```python
from build123d import *

# Parameters (mm, degrees)
F0_W      = 6
F0_H      = 50
F1_DEPTH  = 6
F2_W      = 4
F2_H      = 4
F3_DEPTH  = 5
F5_DEPTH  = 1
F7_DEPTH  = 1
F8_DEPTH  = 4
F10_DEPTH = 25
F11_W     = 1
F11_H     = 4
F12_DEPTH = 25
F13_DEPTH = 15
F14_DEPTH = 15
F16_DEPTH = 1
F18_DEPTH = 1
F20_DEPTH = 4
F21_DEPTH = 1.333
F22_R     = 0.8
F23_SCALE = 0.8


with BuildPart() as f1:
    # F0 (on Top) → F1 (new body)
    with BuildSketch(Plane.XY):
        Rectangle(F0_W, F0_H)
    extrude(amount=F1_DEPTH)

    # F2 (on face) → F3 (join)
    with BuildSketch(Plane.XZ.offset(25)):
        with Locations((0, 2)):
            Rectangle(F2_W, F2_H)
    extrude(amount=F3_DEPTH)

    # F4 (on face) → F5 (cut)
    with BuildSketch(Plane(origin=(-3, 0, 0), x_dir=(0, -1, 0), z_dir=(-1, 0, 0))):
        Polygon((-25, 6), (-25, 0), (-23, 0), align=None)
    extrude(amount=-F5_DEPTH, mode=Mode.SUBTRACT)

    # F6 (on face) → F7 (cut)
    with BuildSketch(Plane.YZ.offset(3)):
        Polygon((23, 0), (25, 0), (25, 6), align=None)
    extrude(amount=-F7_DEPTH, mode=Mode.SUBTRACT)

    # F8 (add): a face of the model
    f8_faces = [f1.faces().sort_by_distance(p)[0] for p in [
        (0, 25, 3),
    ]]
    extrude(f8_faces, amount=F8_DEPTH)

    # F9 (on face) → F10 (cut)
    with BuildSketch(Plane.YZ.offset(2)):
        Polygon((26.5, 4), (26.5, 0), (29, 0), (29, 6), (25, 6), (24.3333333333, 4), align=None)
    extrude(amount=-F10_DEPTH, mode=Mode.SUBTRACT)

    # F11 (on face) → F12 (cut)
    with BuildSketch(Plane(origin=(-2, 0, 0), x_dir=(0, -1, 0), z_dir=(-1, 0, 0))):
        with Locations((29.5, 2)):
            Rectangle(F11_W, F11_H)
    extrude(amount=-F12_DEPTH, mode=Mode.SUBTRACT)

    # F13 (cut): a face of the model
    f13_faces = [f1.faces().sort_by_distance(p)[0] for p in [
        (-2.5, -25, 0.0848528137),
    ]]
    extrude(f13_faces, amount=-F13_DEPTH, mode=Mode.SUBTRACT)

    # F14 (cut): a face of the model
    f14_faces = [f1.faces().sort_by_distance(p)[0] for p in [
        (0, -29, 2),
    ]]
    extrude(f14_faces, amount=-F14_DEPTH, mode=Mode.SUBTRACT)

    # F15 (on face) → F16 (cut)
    with BuildSketch(Plane.YZ.offset(3)):
        Polygon((23, 0), (25, 6), (21, 6), align=None)
    extrude(amount=-F16_DEPTH, mode=Mode.SUBTRACT)

    # F17 (on face) → F18 (cut)
    with BuildSketch(Plane(origin=(-3, 0, 0), x_dir=(0, -1, 0), z_dir=(-1, 0, 0))):
        Polygon((-21, 6), (-25, 6), (-23, 0), align=None)
    extrude(amount=-F18_DEPTH, mode=Mode.SUBTRACT)

    # F19 (on face) → F20 (cut)
    with BuildSketch(Plane(origin=(-2, 0, 0), x_dir=(0, -1, 0), z_dir=(-1, 0, 0))):
        Polygon((-25, 6), (-24.3333333333, 4), (-21.6666666667, 4), (-21, 6), align=None)
    extrude(amount=-F20_DEPTH, mode=Mode.SUBTRACT)

    # F21 (cut): a face of the model
    f21_faces = [f1.faces().sort_by_distance(p)[0] for p in [
        (0, 26.5, 2),
    ]]
    extrude(f21_faces, amount=-F21_DEPTH, mode=Mode.SUBTRACT)

    # F22
    f22_edges = [f1.edges().sort_by_distance(p)[0] for p in [
        (3, 5.5, 6),
        (3, 6.5, 0),
        (-3, 5.5, 6),
        (-3, 6.5, 0),
    ]]
    fillet(f22_edges, radius=F22_R)


with BuildPart() as f1_1:
    # F23: moved
    add(f1.part.scale(F23_SCALE))


solid = f1_1.part
```
Can you work these out from the model? Positions are in its coordinate system, mm. A direction names the side the tool comes from. Coordinates: 2 decimals unless noted, no trailing zeros. Loops run counter-clockwise (first coordinate to the right, second up) from the corner with the lowest first, then second, coordinate; pieces in that order, holes last. Notation, with made-up numbers: (87, -21) -> (92, -21) arc R32 ccw to (92, 6) -> close; hole circle Ø6 at (15.5, -10.5). An arc over 180 degrees is marked (long way). Put each result on its own line as item: value. Start each with the question number.
Q1. I'm going to push flat-ended pins straight in: P1, Ø0.8, axis at x = 0, y = 19.5, coming from the +Z side; P2, Ø1.4, axis at y = 18.5, z = 1.5, coming from the +X side; P3, Ø2.5, axis at y = -9.5, z = 2, coming from the -X side; P4, Ø2.5, axis at y = -10, z = 1, coming from the +X side. Where does each tip first touch, or does it pass through?
Q2. I want a section at B-B (z = 2.4). Write out the boundary of the cut face in (x, y), plus the area to 3 significant figures.
Q3. I want a section at A-A (y = 16.5). Write out the boundary of the cut face in (x, z), plus the area to 3 significant figures.
Q4. I want a section at C-C (x = 0.85). Write out the boundary of the cut face in (y, z), plus the area to 3 significant figures.
Q5. If I drill on line 1 (X direction, y = 2, z = 4.25); line 2 (Z direction, x = 1.1, y = -8.5); line 3 (Z direction, x = -1.8, y = 11.5), over which ranges is the centre line in solid material (lowest first)? Write a range as [from, to].
Q6. For faces 1 (the face through (0, -10, 3.2)), 2 (the face through (0, 19, 3.2)), 3 (the face through (1.6, -10, 2)), which set-ups out of +Z, -Z, +X, -X, +Y, -Y let a thin tool reach every point of the face, with its end or its side?
Taken from the geometry:
1. P1: stops at z = 3.2
1. P2: stops at x = 2.4
1. P3: stops at x = -1.6
1. P4: stops at x = 1.6
2. outline: (-2.4, -8) -> (-1.6, -8) -> (-1.6, -11.2) -> (1.6, -11.2) -> (1.6, -8) -> (2.4, -8) -> (2.4, 17.6) -> (1.6, 17.6) -> (1.6, 20.13) -> (-1.6, 20.13) -> (-1.6, 17.6) -> (-2.4, 17.6) -> close
2. area: 141 mm2
3. outline: (-2.4, 0.64) arc R0.64 ccw to (-1.76, 0) -> (1.76, 0) arc R0.64 ccw to (2.4, 0.64) -> (2.4, 4.16) arc R0.64 ccw to (1.76, 4.8) -> (-1.76, 4.8) arc R0.64 ccw to (-2.4, 4.16) -> close
3. area: 22.7 mm2
4. outline: (-11.2, 0) -> (20.13, 0) -> (20.13, 3.2) -> (17.33, 3.2) -> (16.8, 4.8) -> (-8, 4.8) -> (-8, 3.2) -> (-11.2, 3.2) -> close
4. area: 140 mm2
5. line 1: x = [-2.39, 2.39]
5. line 2: z = [0, 3.2]
5. line 3: z = [0, 4.8]
6. face 1: +Z, +X, -X, -Y
6. face 2: +Z, +X, -X, +Y
6. face 3: +Z, -Z, +X, -Y
